The model under review builds one solid part; all positions refer to its coordinate system, in mm. Face numbers are marked on the shaded views. A direction names the side the tool comes from. Give positions to 0.01 mm unless a question says otherwise; leave off trailing zeros. Order: outer loops, then holes, each group sorted by start corner. A loop starts at its lowest first (then second) coordinate and runs counter-clockwise, first axis right, second up. Notation, with made-up numbers: (31, 10.25) - (88, 10.25) arc R9 cw to (88, 15.25) - close; hole circle Ø10 at (40, 10). An arc over 180 degrees is marked (long way). Use CSV: the item, a comma, the result in double quotes. Start each with the question number.
1. Take a section at C-C, the plane y = 45.5. State the section outline as (x, z) points.
2. To check wall thickness, follow line 1 (Y direction, x = 0, z = -6.9); line 2 (Y direction, x = -1.5, z = -9.5); line 3 (Z direction, x = -2, y = 43.5). State the ranges of each line that lie inside material, in increasing order. Write a range as [from, to].
3. Machinability: for the marked faces 4 and 5, which of the approach directions +Z, -Z, +X, -X, +Y, -Y give a long, thin tool a straight path to every point of the face, cutting with its end or side? Answer none if there is none.
4. Take a section at B-B, the plane z = -5.75. State the section outline as (x, y) points, then the cut area to 3 significant figures.
5. Take a section at A-A, the plane x = 0. State the section outline as (y, z) points.
6. Take a section at D-D, the plane y = 48. State the section outline as (x, z) points, then the cut area to 3 significant figures.
7. For pin 1 (3 mm diameter, centred on x = -1, z = -3, fed in from -Y); pin 2 (4 mm diameter, centred on y = 45.5, z = -2.5, fed in from +X); pin 3 (0.9 mm diameter, centred on x = -0.5, y = 48, fed in from +Z); pin 4 (1 mm diameter, centred on x = -2, y = 44, fed in from -Z), all flat-tipped, find the tip position at first contact; note any pin that passes through.
8. Draft analysis for pull direction Y (two halves, no side actions). For the marked faces 1, 2 and 3, state which applies: released by +Y, released by -Y, zero draft, split by the parting line, or undercut.
```python
from build123d import *

# Parameters (mm, degrees)
CROQUIS1_R              = 4
SALIENTE_EXTRUIR1_DEPTH = 10
CROQUIS2_W              = 2
CROQUIS2_H              = 13.059807194
CORTAR_EXTRUIR1_DEPTH   = 6
CROQUIS3_R              = 3
CORTAR_EXTRUIR2_DEPTH   = 5


with BuildPart() as part:
    # Croquis1 → Saliente-Extruir1 (new body)
    with BuildSketch(Plane.XY):
        with Locations((0, 44.649122807)):
            Circle(CROQUIS1_R)
    extrude(amount=-SALIENTE_EXTRUIR1_DEPTH)

    # Croquis2 → Cortar-Extruir1 (cut)
    with BuildSketch(Plane.XY):
        with Locations((0, 44.649122807)):
            Rectangle(CROQUIS2_W, CROQUIS2_H)
    extrude(amount=-CORTAR_EXTRUIR1_DEPTH, mode=Mode.SUBTRACT)

    # Croquis3 → Cortar-Extruir2 (cut)
    with BuildSketch(Plane(origin=(0, 0, -10), x_dir=(-1, 0, 0), z_dir=(0, 0, -1))):
        with Locations((0, 44.649122807)):
            Circle(CROQUIS3_R)
    extrude(amount=-CORTAR_EXTRUIR2_DEPTH, mode=Mode.SUBTRACT)


solid = part.part
```
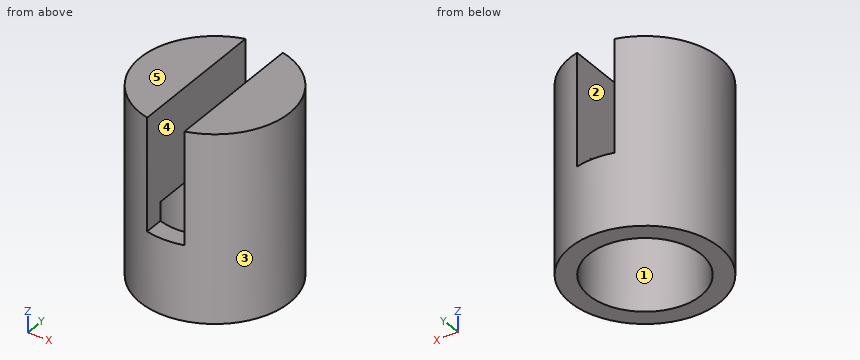
Determined:
1,outline,"(-3.91, -10) - (-2.88, -10) - (-2.88, -5) - (-1, -5) - (-1, 0) - (-3.91, 0) - close; (1, -5) - (2.88, -5) - (2.88, -10) - (3.91, -10) - (3.91, 0) - (1, 0) - close"
2,line 1,"y = [40.65, 41.65], [47.65, 48.65]"
2,line 2,"y = [40.94, 42.05], [47.25, 48.36]"
2,line 3,"z = [-5, 0]"
3,face 4,"+Z, +Y, -Y"
3,face 5,"+Z, +X, -X, +Y, -Y"
4,outline,"(-1, 40.78) - (-1, 41.82) arc R3 cw to (-1, 47.48) - (-1, 48.52) arc R4 ccw to start; (1, 40.78) arc R4 ccw to (1, 48.52) - (1, 47.48) arc R3 cw to (1, 41.82) - close"
4,area,"17.9 mm²"
5,outline,"(40.65, -10) - (41.65, -10) - (41.65, -6) - (40.65, -6) - close; (47.65, -10) - (48.65, -10) - (48.65, -6) - (47.65, -6) - close"
6,outline,"(-2.18, -10) - (2.18, -10) - (2.18, 0) - (1, 0) - (1, -6) - (-1, -6) - (-1, 0) - (-2.18, 0) - close"
6,area,"31.7 mm²"
7,pin 1,"stops at y = 40.78"
7,pin 2,"stops at x = 4"
7,pin 3,"stops at z = -6"
7,pin 4,"stops at z = -5"
8,face 1,"undercut"
8,face 2,"zero draft"
8,face 3,"split by the parting line"
